Input: dimensioned drawing with shaded views. Units: mm. Origin: part minimum x, y, z. A direction names the side the tool comes from. Round coordinates to 2 decimals unless told otherwise and drop trailing zeros. Write each loop counter-clockwise with the first axis right and the second up, starting at its lowest first coordinate (ties: lowest second). Pieces come first, ordered by that corner, then holes. Notation, with made-up numbers: (62.5, -7.75) -> (75.5, -7.75) arc R21 ccw to (75.5, 8.25) -> close; hole circle Ø8 at (22, 78). An arc over 180 degrees is marked (long way). Use one line per item in the form item = value. Start each with the question number.
1. Line query: L1, parallel to X at y = 1.25, z = 12; L2, parallel to Z at x = 20, y = 3.2 (1 decimal); L3, parallel to X at y = 4, z = 1.5 (1 decimal). Output: solid intervals per line, ascending.
2. Cut plane A-A, the plane z = 12. State how many separate pieces and enclosed holes the cut face has.
3. Reachability of the marked faces 4, 5 and 6 from +Z, -Z, +X, -X, +Y, -Y: full face, straight path, thin tool, end or side. Return the list, or none.
4. Draft query along Z for the marked faces 1, 2 and 3. Return one class per face: pulls with the +Z half, pulls with the -Z half, needs draft (parallel to the pull), parting line crosses it, or undercut.
5. Cut plane D-D, the plane y = 0.95. Return the cut outline in (x, z).
6. Pin query (flat end, axial travel): pin 1 Ø4 at (x, z) = (12, 12) entering from +Y; pin 2 Ø1.7 at (x, z) = (9.61, 18.58) entering from -Y; pin 3 Ø1.5 at (x, y) = (5.5, 2) entering from -Z (1 decimal). Return the tip coordinate at first contact, or that it passes through.
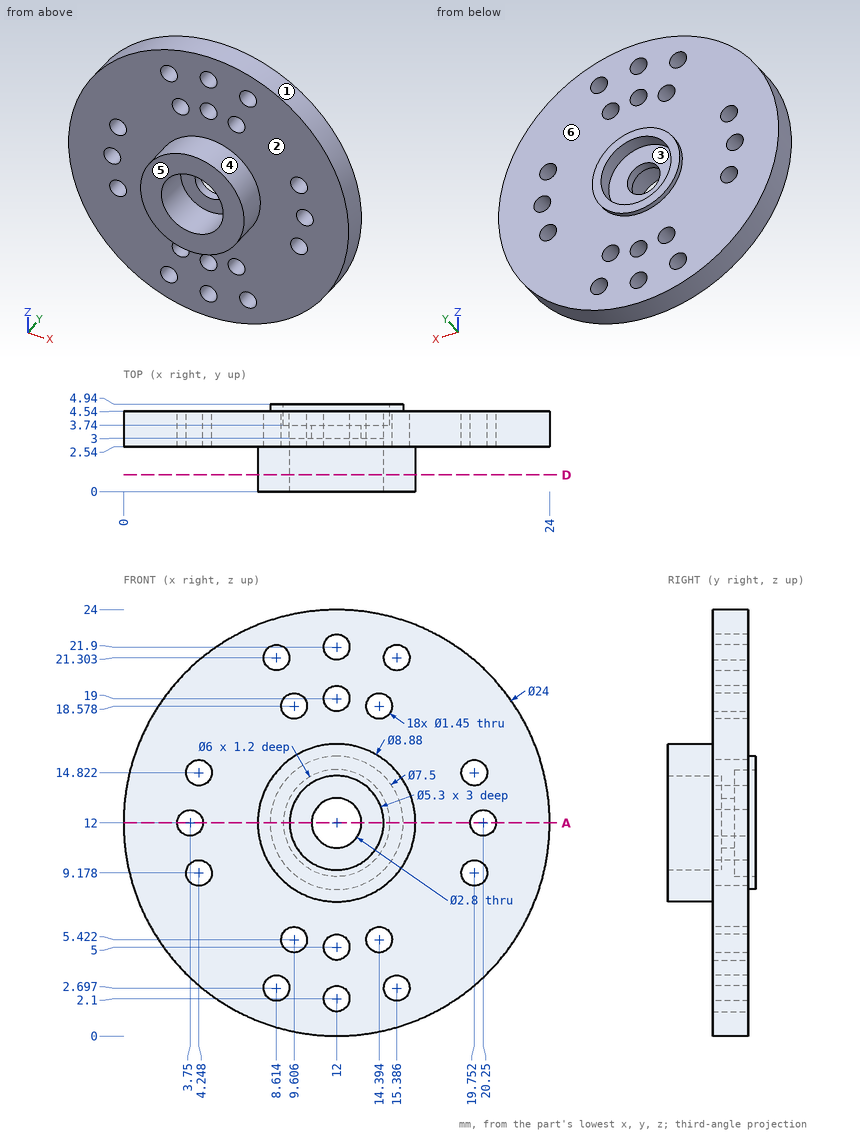
Outcome:
q1.L1 = 7.56 to 9.35, 14.65 to 16.44
q1.L2 = 3.1 to 8.5, 9.9 to 11.3, 12.7 to 14.1, 15.5 to 20.9
q1.L3 = 6.2 to 11.6, 12.4 to 17.8
q2.separate_pieces = 4
q2.enclosed_holes = 0
q3.face_4 = -Y
q3.face_5 = +Z, -Z, +X, -X, -Y
q3.face_6 = +Y
q4.face_1 = parting line crosses it
q4.face_2 = needs draft
q4.face_3 = undercut
q5.outline = circle Ø8.88 at (12, 12); hole circle Ø5.3 at (12, 12)
q6.pin_1 = 3.74
q6.pin_2 = 2.54
q6.pin_3 = 1.6
